Drawing for the job (mm, zero at the part's lowest x, y, z). A direction names the side the tool comes from. Round coordinates to 2 decimals unless told otherwise and drop trailing zeros. Order: outer loops, then holes, each group sorted by start corner. A loop starts at its lowest first (then second) coordinate and runs counter-clockwise, first axis right, second up. Notation, with made-up numbers: (-9.75, 4.5) - (1.25, 4.5) arc R11 cw to (1.25, 15.5) - close; hole circle Ø2 at (20.25, -35). An arc over 180 degrees is marked (long way). Put each result on its own line as item: value. Start each with the question number.
Item 1: Which spindle directions (+Z, -Z, +X, -X, +Y, -Y) get a long thin tool onto all of the face, cutting with end or side? Do the marked faces 1, 2, 3 and 4. Say none if no direction does.
Item 2: Mould opens along Z. For the marked faces 5, 6 and 7 say: pulls with the +Z half, pulls with the -Z half, needs draft (parallel to the pull), parting line crosses it, or undercut.
Item 3: Pin check, flat tips, straight feed: pin 1 Ø5 at (y, z) = (5, 6.5) entering from -X; pin 2 Ø1.5 at (x, z) = (7.5, 1.5) entering from +Y; pin 3 Ø1.5 at (x, y) = (3.5, 10.5) entering from +Z. Stop position of each tip, or through.
Item 4: Saw through at D-D on y = 10.25. List the corners of the cut face in (x, z), plus the area to 3 significant figures.
Item 5: Saw through at C-C on x = 14.25. List the corners of the cut face in (y, z), plus the area to 3 significant figures.
Item 6: Probe probe 1 along X at (y, z) = (0.5, 4.25); probe 2 along Z at (x, y) = (12.75, 5.85); probe 3 along Z at (x, y) = (5.5, 4). List the from-to ranges inside material, lowest first.
Item 7: Saw through at A-A on y = 5.85. List the corners of the cut face in (x, z).
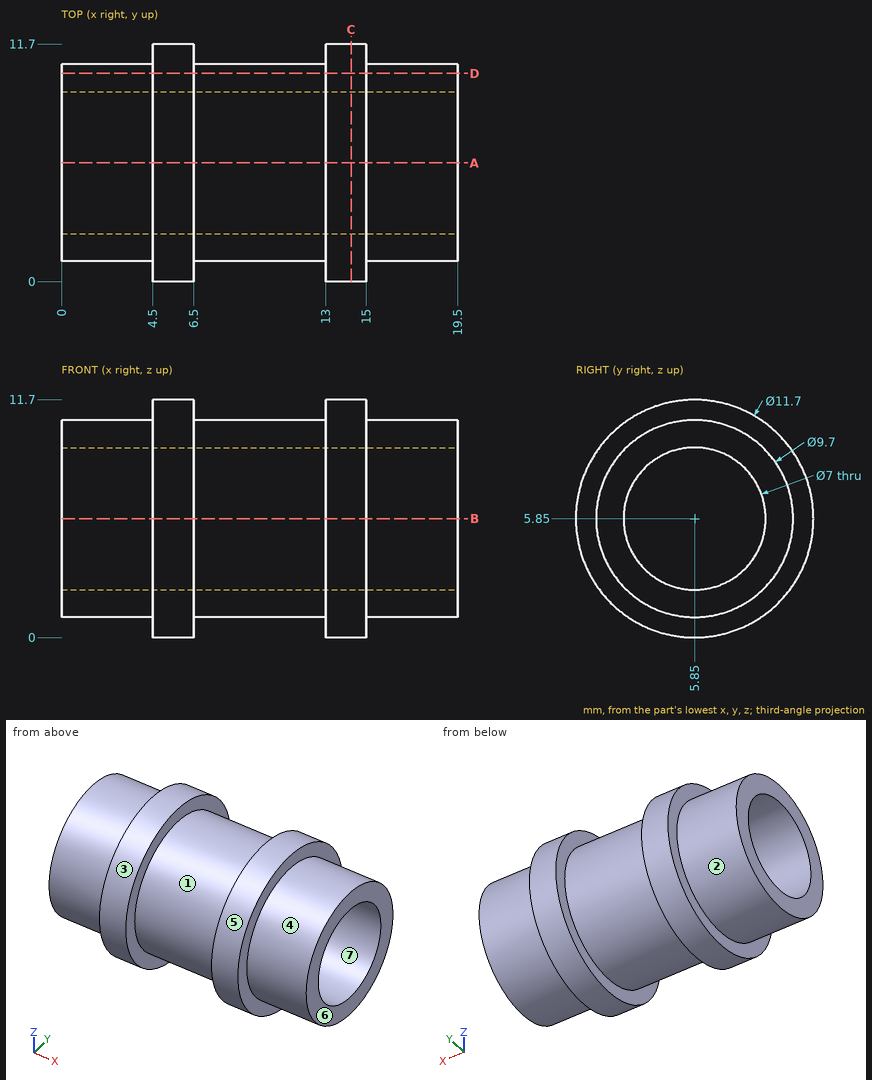
Results found:
1. face 1: none
1. face 2: -X
1. face 3: +X, -X
1. face 4: +X
2. face 5: parting line crosses it
2. face 6: needs draft
2. face 7: undercut
3. pin 1: stops at x = 0
3. pin 2: stops at y = 9.1
3. pin 3: stops at z = 8.73
4. outline: (0, 3.81) - (4.5, 3.81) - (4.5, 1.99) - (6.5, 1.99) - (6.5, 3.81) - (13, 3.81) - (13, 1.99) - (15, 1.99) - (15, 3.81) - (19.5, 3.81) - (19.5, 7.89) - (15, 7.89) - (15, 9.71) - (13, 9.71) - (13, 7.89) - (6.5, 7.89) - (6.5, 9.71) - (4.5, 9.71) - (4.5, 7.89) - (0, 7.89) - close
4. area: 94.1 mm²
5. outline: circle Ø11.7 at (5.85, 5.85); hole circle Ø7 at (5.85, 5.85)
5. area: 69.0 mm²
6. probe 1: x = 4.5 to 6.5, 13 to 15
6. probe 2: z = 1 to 2.35, 9.35 to 10.7
6. probe 3: z = 0.3 to 2.88, 8.82 to 11.4
7. outline: (0, 1) - (4.5, 1) - (4.5, 0) - (6.5, 0) - (6.5, 1) - (13, 1) - (13, 0) - (15, 0) - (15, 1) - (19.5, 1) - (19.5, 2.35) - (0, 2.35) - close; (0, 9.35) - (19.5, 9.35) - (19.5, 10.7) - (15, 10.7) - (15, 11.7) - (13, 11.7) - (13, 10.7) - (6.5, 10.7) - (6.5, 11.7) - (4.5, 11.7) - (4.5, 10.7) - (0, 10.7) - close
